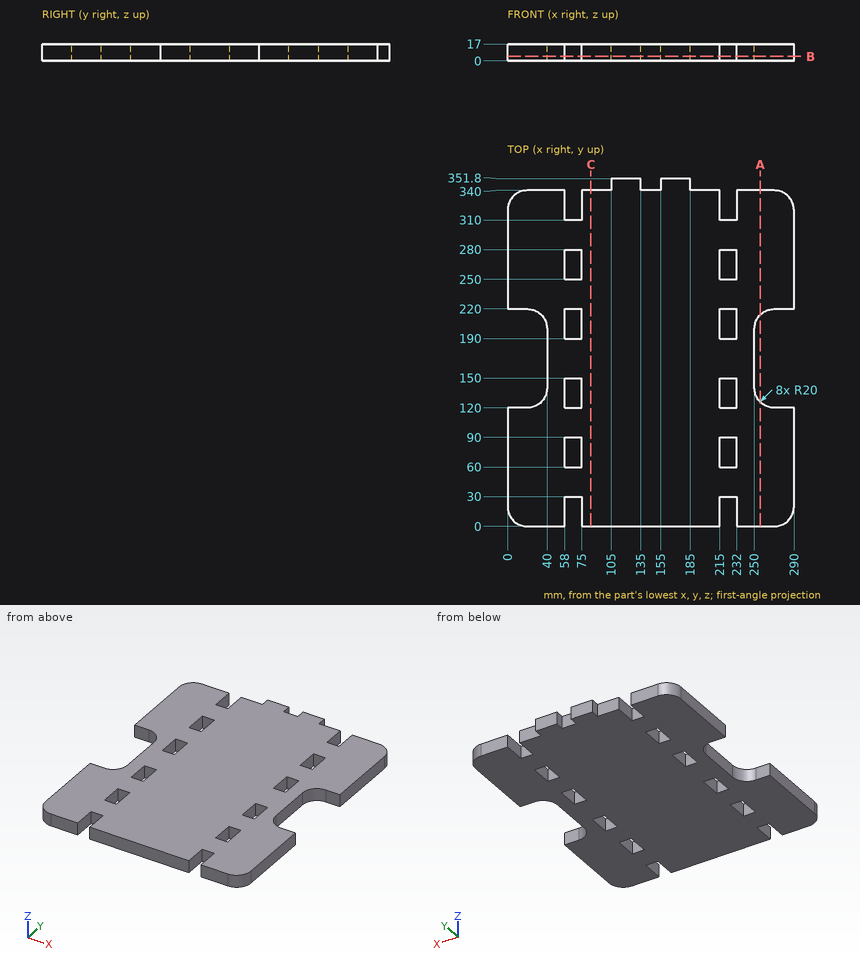
The figure shows three views and two pictorial views of one solid part (mm, origin at its lowest corner). Answer the questions. Round coordinates to 2 decimals unless told otherwise and drop trailing zeros. Loops run counter-clockwise (first coordinate to the right, second up) from the corner with the lowest first, then second, coordinate; pieces in that order, holes last. Notation, with made-up numbers: (40, 62) - (59, 62) arc R32 ccw to (59, 97) - close; hole circle Ø4 at (73.5, 47.5). An arc over 180 degrees is marked (long way). Use one line per item in the form item = value. Start each with the question number.
(1) Find section B-B on z = 4.5. Give the number of separate pieces and of enclosed holes in the cut face, and give its area (3 significant figures).
(2) Flat-ended cylindrical pins translate along their axes: P1, Ø5, axis at y = 266, z = 8, coming from the -X side; P2, Ø5, axis at y = 11.5, z = 8.5, coming from the -X side; P3, Ø8.5, axis at y = 211, z = 12, coming from the -X side; P4, Ø8.5, axis at x = 63, z = 10, coming from the -Y side. Find the tip coordinate at first contact, or state that the pin passes through.
(3) Consider line 1 (Y direction, x = 231.5, z = 9.5); line 2 (X direction, y = 311, z = 10.5); line 3 (X direction, y = 121.5, z = 9.75). Determine where each line is inside the solid, lowest interval first.
(4) Find section C-C on x = 84.5. Determine the outline of the cut face in (y, z).
(5) Find section A-A on x = 256. Determine the outline of the cut face in (y, z).
Answer list:
q1.separate_pieces = 1
q1.enclosed_holes = 8
q1.area = 85,200 mm^2
q2.P1 = 0
q2.P2 = 0.92
q2.P3 = 32.94
q2.P4 = 30
q3.line_1 = 30 to 60, 90 to 120, 150 to 190, 220 to 250, 280 to 310
q3.line_2 = 0 to 58, 75 to 215, 232 to 290
q3.line_3 = 27.6 to 58, 75 to 215, 232 to 262.4
q4.outline = (0, 0) - (340, 0) - (340, 17) - (0, 17) - close
q5.outline = (0, 0) - (125.72, 0) - (125.72, 17) - (0, 17) - close; (214.28, 0) - (340, 0) - (340, 17) - (214.28, 17) - close
